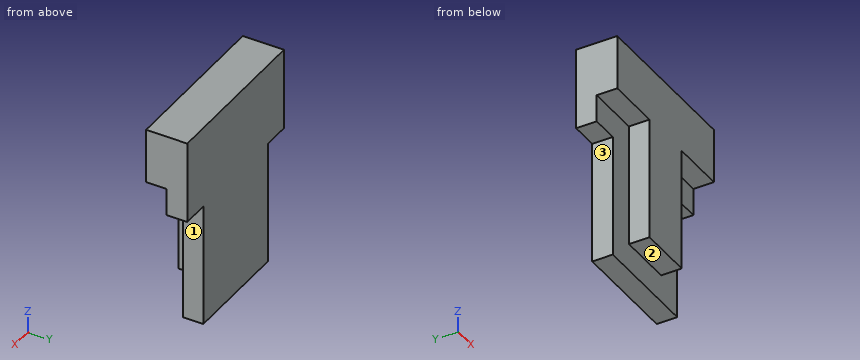
```python
from build123d import *

# Parameters (mm, degrees)
F1_DEPTH = 7.62
F2_DEPTH = 3.81


# Not quite as in the source:
# - a feature names something its author has since deleted; it is built from what else it names


with BuildPart() as f1:
    # F0 (on Front) → F1 (new body)
    with BuildSketch(Plane.XZ):
        Polygon((-20.32, 5.08), (-20.32, -17.78), (-10.16, -17.78), (-10.16, 5.08), (0, 5.08), (0, 15.24), (-30.48, 15.24), (-30.48, 5.08), align=None)
    extrude(amount=F1_DEPTH)

    # F0 (on Front) → F2 (join)
    with BuildSketch(Plane.XZ):
        Polygon((-10.16, 5.08), (-10.16, -17.78), (-5.08, -17.78), (-5.08, 0), (0, 0), (0, 5.08), align=None)
        Polygon((-20.32, -17.78), (-25.4, -17.78), (-25.4, -22.86), (-5.08, -22.86), (-5.08, -17.78), (-10.16, -17.78), align=None)
        Polygon((-25.4, 0), (-25.4, -17.78), (-20.32, -17.78), (-20.32, 5.08), (-30.48, 5.08), (-30.48, 0), align=None)
    extrude(amount=F2_DEPTH)


solid = f1.part
```
The model under review builds one solid part; all positions refer to its coordinate system, in mm. Face numbers are marked on the shaded views. A direction names the side the tool comes from. Coordinates: 2 decimals unless noted, no trailing zeros. Write each loop counter-clockwise with the first axis right and the second up, starting at its lowest first coordinate (ties: lowest second). Pieces come first, ordered by that corner, then holes. Notation, with made-up numbers: (-1, 78) - (39, 78) arc R9 ccw to (39, 88) - close; hole circle Ø3 at (48, 47.25). An arc over 180 degrees is marked (long way). Answer in a Markdown table with one row per item. Add a question column.
Q1. Clearance check with flat-ended pins moving along their axes: pin 1 (1 mm diameter, centred on x = -11.5, z = 3.5, fed in from +Y); pin 2 (4 mm diameter, centred on y = -1.5, z = -6, fed in from -X); pin 3 (1.9 mm diameter, centred on x = -26.5, y = -6.5, fed in from -Z); pin 4 (1.1 mm diameter, centred on x = -27.5, y = -1, fed in from -Z). State where each tip first meets the part, or that it passes through.
Q2. Consider section B-B on x = -7. Give the boundary of the cut face in (y, z), then the cut area to 3 significant figures.
Q3. To check wall thickness, follow line 1 along Y through (x, z) = (-7, 4.5); line 2 along X through (y, z) = (-3.75, -2); line 3 along X through (y, z) = (-7, 1). State the ranges of each line that lie inside material, in increasing order. Write a range as from..to.
Q4. For the marked faces 1, 2 and 3, list the 3-axis set-ups (+Z, -Z, +X, -X, +Y, -Y) from which the entire face can be reached by the end or side of a thin tool; tool diameter is ignored.
Q5. Consider section C-C on y = -2.5. Give the boundary of the cut face in (x, z).
Q6. Consider section D-D on x = -12. Give the boundary of the cut face in (y, z).
Q7. Consider section A-A on z = -7.5. Give the boundary of the cut face in (x, y).
Answers below:
| question | item | result |
|---|---|---|
| 1 | pin 1 | y = 0 |
| 1 | pin 2 | x = -25.4 |
| 1 | pin 3 | z = 5.08 |
| 1 | pin 4 | z = 0 |
| 2 | outline | (-7.62, 5.08) - (-3.81, 5.08) - (-3.81, -22.86) - (0, -22.86) - (0, 15.24) - (-7.62, 15.24) - close |
| 2 | area | 184 mm² |
| 3 | line 1 | -3.81..0 |
| 3 | line 2 | -25.4..-5.08 |
| 3 | line 3 | -20.32..-10.16 |
| 4 | face 1 | -Z, +X, +Y, -Y |
| 4 | face 2 | -Z, +X, -X, -Y |
| 4 | face 3 | -Z, -X, +Y, -Y |
| 5 | outline | (-30.48, 0) - (-25.4, 0) - (-25.4, -22.86) - (-5.08, -22.86) - (-5.08, 0) - (0, 0) - (0, 15.24) - (-30.48, 15.24) - close |
| 6 | outline | (-7.62, -17.78) - (-3.81, -17.78) - (-3.81, -22.86) - (0, -22.86) - (0, 15.24) - (-7.62, 15.24) - close |
| 7 | outline | (-25.4, -3.81) - (-20.32, -3.81) - (-20.32, -7.62) - (-10.16, -7.62) - (-10.16, -3.81) - (-5.08, -3.81) - (-5.08, 0) - (-25.4, 0) - close |
